Geometry check sheet. Reference: the model listing, model coordinates, mm. A direction names the side the tool comes from. Round coordinates to 2 decimals unless told otherwise and drop trailing zeros. Loops run counter-clockwise (first coordinate to the right, second up) from the corner with the lowest first, then second, coordinate; pieces in that order, holes last. Notation, with made-up numbers: M 35,-13.5 L 47,-13.5 A16 ccw 47,5.5 Z; hole C 2,11 d8. An arc over 180 degrees is marked long. Answer in a Markdown table with one row per item. Add a question column.
```python
from build123d import *

# Parameters (mm, degrees)
EXTRUDE_1_DEPTH     = 55
EXTRUDE_2_DEPTH     = 10
SKETCH_3_W          = 15
SKETCH_3_H          = 15
CUT_EXTRUDE_1_DEPTH = 99.234413522
CUT_EXTRUDE_START   = -8
CUT_EXTRUDE_2_DEPTH = 12


with BuildPart() as part:
    # Эскиз1 → Бобышка-Вытянуть1 (new body)
    with BuildSketch(Plane.XY):
        Polygon((-20, 27.5), (-20, 12.5), (-3, 12.5), (-3, -27.5), (20, -27.5), (5, -14.913505532), (5, 27.5), align=None)
    extrude_1 = extrude(amount=EXTRUDE_1_DEPTH)

    # Эскиз2 → Бобышка-Вытянуть2 (add)
    with BuildSketch(Plane(origin=(0, 0, 0), x_dir=(-1, 0, 0), z_dir=(0, 0, -1))):
        Polygon((-5, 27.5), (-20, -27.5), (-5, -14.913505532), align=None)
    extrude_2 = extrude(amount=-EXTRUDE_2_DEPTH)

    # Зеркальное отражение1: Бобышка-Вытянуть1, Бобышка-Вытянуть2 across plane
    add(extrude_1.mirror(Plane(origin=(-20, 0, 55), x_dir=(0, 0, 1), z_dir=(-1, 0, 0))))
    add(extrude_2.mirror(Plane(origin=(-20, 0, 55), x_dir=(0, 0, 1), z_dir=(-1, 0, 0))))

    # Эскиз3 → Вырез-Вытянуть1 (cut, through all)
    with BuildSketch(Plane(origin=(0, 27.5, 0), x_dir=(1, 0, 0), z_dir=(0, 1, 0))):
        with Locations((-14.5, -17.5)):
            Rectangle(SKETCH_3_W, SKETCH_3_H)
    extrude(amount=-CUT_EXTRUDE_1_DEPTH, mode=Mode.SUBTRACT)

    # Эскиз4 → Вырез-Вытянуть2 (cut)
    with BuildSketch(Plane.XY.offset(55).offset(CUT_EXTRUDE_START)):
        Polygon((-45, 27.5), (-45, 13.5), (-31, 27.5), align=None)
    extrude(amount=-CUT_EXTRUDE_2_DEPTH, mode=Mode.SUBTRACT)


solid = part.part
```
1) Cross-section at C-C, the plane y = -6. Record the boundary of the cut face in (x, z), plus the area to 3 significant figures.
2) Cross-section at A-A, the plane x = -8. Record the boundary of the cut face in (y, z).
3) Go/stop test with flat-tipped pins: pin 1 (1.5 mm diameter, centred on y = 5, z = 14, fed in from -X); pin 2 (12 mm diameter, centred on y = -14, z = 30, fed in from +X); pin 3 (10 mm diameter, centred on x = -7.5, z = 9.5, fed in from -Y); pin 4 (16.5 mm diameter, centred on y = 20.5, z = 18, fed in from -X). Record where each tip stops, or that it passes through.
4) Draft check along X on faces 1 (the flat face through (-21, 13, 0)), 2 (the flat face through (-37, -7, 27)), 3 (the flat face through (-22, 20, 18)), 4 (the flat face through (12.395, 0.385, 4.93)). Enter one of: +X half, -X half, draft (parallel to the pull), parting line (faces both ways), or undercut.
5) Cross-section at B-B, the plane z = 13. Record the boundary of the cut face in (x, y).
6) Cross-section at D-D, the plane x = -34. Record the boundary of the cut face in (y, z), plus the area to 3 significant figures.
7) Thickness scan on L1, parallel to X at y = -6.5, z = 36.5; L2, parallel to X at y = 13, z = 19; L3, parallel to Z at x = -15, y = 16. Record the ranges inside material, lowest first. Write a range as [from, to].
8) Set-up check for faces 5 (the flat face through (-15, 20, 25)), 6 (the flat face through (-40, 22, 35)), 7 (the flat face through (10, -6, 10)), 8 (the flat face through (-52.6, -21.29, 32.18)), 9 (the flat face through (-3, -7, 27)): record each of +Z, -Z, +X, -X, +Y, -Y from which the full face is reachable in a straight line by a thin tool's end or side.
Worked answers:
| question | item | result |
|---|---|---|
| 1 | outline | M -54.14,0 L -37,0 L -37,55 L -45,55 L -45,10 L -54.14,10 Z; M -3,0 L 14.14,0 L 14.14,10 L 5,10 L 5,55 L -3,55 Z |
| 1 | area | 1,060 mm2 |
| 2 | outline | M 12.5,0 L 27.5,0 L 27.5,10 L 12.5,10 Z; M 12.5,25 L 27.5,25 L 27.5,55 L 12.5,55 Z |
| 3 | pin 1 | stops at x = -45 |
| 3 | pin 2 | stops at x = 11.06 |
| 3 | pin 3 | stops at y = -27.5 |
| 3 | pin 4 | stops at x = -47.46 |
| 4 | face 1 | draft |
| 4 | face 2 | undercut |
| 4 | face 3 | undercut |
| 4 | face 4 | +X half |
| 5 | outline | M -60,-27.5 L -37,-27.5 L -37,12.5 L -22,12.5 L -22,27.5 L -45,27.5 L -45,-14.91 Z; M -7,12.5 L -3,12.5 L -3,-27.5 L 20,-27.5 L 5,-14.91 L 5,27.5 L -7,27.5 Z |
| 6 | outline | M 12.5,0 L 27.5,0 L 27.5,35 L 24.5,35 L 24.5,47 L 27.5,47 L 27.5,55 L 12.5,55 Z |
| 6 | area | 789 mm2 |
| 7 | L1 | x = [-45, -37], [-3, 5] |
| 7 | L2 | x = [-45, -22], [-7, 5] |
| 7 | L3 | z = [0, 10], [25, 55] |
| 8 | face 5 | +Y, -Y |
| 8 | face 6 | -X, +Y |
| 8 | face 7 | +Z, +X, +Y |
| 8 | face 8 | +Z, -X, +Y |
| 8 | face 9 | +Z, -Z, -Y |
